```python
from build123d import *

# Parameters (mm, degrees)
SKETCH1_W           = 130
SKETCH1_H           = 190
BOSS_EXTRUDE1_DEPTH = 5
SKETCH2_W           = 130
SKETCH2_H           = 190
SKETCH2_W_2         = 120
SKETCH2_H_2         = 180
BOSS_EXTRUDE2_DEPTH = 130
BOSS_EXTRUDE3_DEPTH = 10
SKETCH4_W           = 2.4
SKETCH4_H           = 5
CUT_EXTRUDE1_DEPTH  = 187.4
SKETCH5_W           = 120
SKETCH5_H           = 5
CUT_EXTRUDE2_DEPTH  = 2.4


with BuildPart() as part:
    # Sketch1 → Boss-Extrude1 (new body)
    with BuildSketch(Plane.XY):
        with Locations((65, -95)):
            Rectangle(SKETCH1_W, SKETCH1_H)
    extrude(amount=BOSS_EXTRUDE1_DEPTH)

    # Sketch2 → Boss-Extrude2 (add)
    with BuildSketch(Plane.XY.offset(5)):
        with Locations((65, -95)):
            Rectangle(SKETCH2_W, SKETCH2_H)
        with Locations((65, -95)):
            Rectangle(SKETCH2_W_2, SKETCH2_H_2, mode=Mode.SUBTRACT)
    extrude(amount=BOSS_EXTRUDE2_DEPTH)

    # Sketch3 → Boss-Extrude3 (add)
    with BuildSketch(Plane.XY.offset(135)):
        Polygon((0, -190), (0, 0), (130, 0), (130, -190), (125, -190), (125, -185), (125, -5), (5, -5), (5, -190), align=None)
    extrude(amount=BOSS_EXTRUDE3_DEPTH)

    # Sketch4 → Cut-Extrude1 (cut)
    with BuildSketch(Plane.XZ.offset(190)):
        with Locations((3.8, 137.5)):
            Rectangle(SKETCH4_W, SKETCH4_H)
        with Locations((126.2, 137.5)):
            Rectangle(SKETCH4_W, SKETCH4_H)
    extrude(amount=-CUT_EXTRUDE1_DEPTH, mode=Mode.SUBTRACT)

    # Sketch5 → Cut-Extrude2 (cut)
    with BuildSketch(Plane.XZ.offset(5)):
        with Locations((65, 137.5)):
            Rectangle(SKETCH5_W, SKETCH5_H)
    extrude(amount=-CUT_EXTRUDE2_DEPTH, mode=Mode.SUBTRACT)


solid = part.part
```
Could you check a few things on this model? Use its own coordinates, in mm. A direction names the side the tool comes from. Coordinates: 2 decimals unless noted, no trailing zeros. Write each loop counter-clockwise with the first axis right and the second up, starting at its lowest first coordinate (ties: lowest second). Pieces come first, ordered by that corner, then holes. Notation, with made-up numbers: (-18, 25.25) -> (7, 25.25) arc R9 ccw to (7, 34.25) -> close; hole circle Ø3 at (54, 71). An arc over 180 degrees is marked (long way). Return JSON: item names as keys, results as strings.
(1) Imagine slicing it at A-A, the plane z = 69. Please give me the cut outline in (x, y), then the cut area to 3 significant figures.
Numbers:
{"outline": "(0, -190) -> (130, -190) -> (130, 0) -> (0, 0) -> close; hole (5, -185) -> (125, -185) -> (125, -5) -> (5, -5) -> close", "area": "3,100 mm2"}
(2) I need wall thicknesses on L1, parallel to Y at x = 22.5, z = 112; L2, parallel to X at y = -22.5, z = 116; L3, parallel to Z at x = 43, y = -126. Which ranges of each line are inside material? Lowest first, please.
Numbers:
{"L1": "y = -190 to -185, -5 to 0", "L2": "x = 0 to 5, 125 to 130", "L3": "z = 0 to 5"}
(3) Imagine slicing it at C-C, the plane y = -171. Please give me the cut outline in (x, z).
Numbers:
{"outline": "(0, 0) -> (130, 0) -> (130, 145) -> (125, 145) -> (125, 140) -> (127.4, 140) -> (127.4, 135) -> (125, 135) -> (125, 5) -> (5, 5) -> (5, 135) -> (2.6, 135) -> (2.6, 140) -> (5, 140) -> (5, 145) -> (0, 145) -> close"}
(4) I'm going to push flat-ended pins straight in: pin 1 (10 mm diameter, centred on x = 115.5, y = -33.5, fed in from +Z); pin 2 (4 mm diameter, centred on x = 37, z = 143, fed in from -Y). Where does each tip first touch, or does it pass through?
Numbers:
{"pin 1": "stops at z = 5", "pin 2": "stops at y = -5"}
(5) Which directions (+Z, -Z, +X, -X, +Y, -Y) give clear straight access to the entire face, cutting with the end or side of a thin tool? Please do faces 4 (the flat face through (64, -94, 0)), 5 (the flat face through (66, -5, 69)), 6 (the flat face through (125, -96, 142)), 7 (the flat face through (64, -2.6, 138)).
Numbers:
{"face 4": "-Z, +X, -X, +Y, -Y", "face 5": "+Z", "face 6": "+Z, -Y", "face 7": "-Y"}
(6) Imagine slicing it at B-B, the plane x = 85. Please give me the cut outline in (y, z).
Numbers:
{"outline": "(-190, 0) -> (0, 0) -> (0, 145) -> (-5, 145) -> (-5, 140) -> (-2.6, 140) -> (-2.6, 135) -> (-5, 135) -> (-5, 5) -> (-185, 5) -> (-185, 135) -> (-190, 135) -> close"}
(7) We'd pull the mould along Z, two halves only. Please class faces 1 (the flat face through (125, -94, 69)), 2 (the flat face through (64, -94, 5)), 3 (the flat face through (4.6, -137.5, 135)): +Z half, -Z half, draft (parallel to the pull), parting line (faces both ways), or undercut.
Numbers:
{"face 1": "draft", "face 2": "+Z half", "face 3": "undercut"}
